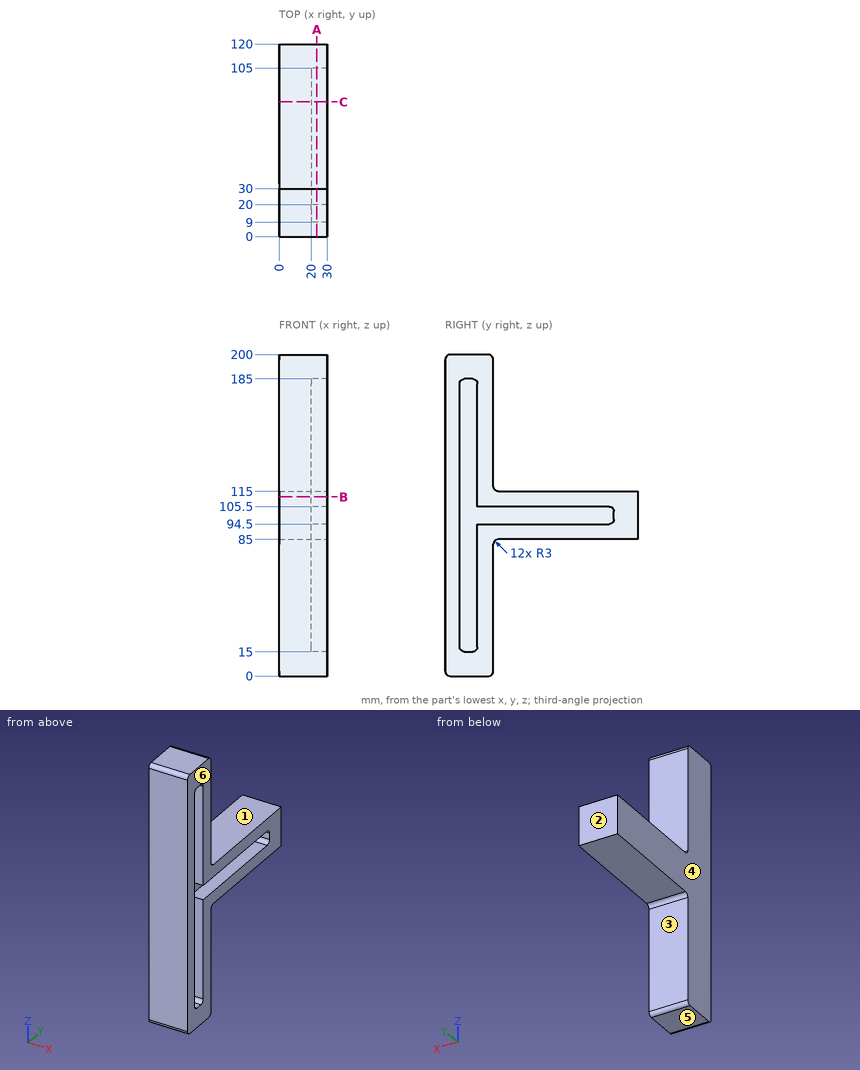
Check sheet for the drawn part. Datum: minimum x, y, z corner. Units: mm. A direction names the side the tool comes from. Round coordinates to 2 decimals unless told otherwise and drop trailing zeros. Loops run counter-clockwise (first coordinate to the right, second up) from the corner with the lowest first, then second, coordinate; pieces in that order, holes last. Notation, with made-up numbers: (12, 7) - (46, 7) arc R38 cw to (46, 45) - close; hole circle Ø3 at (77.25, 86.5). An arc over 180 degrees is marked (long way). Answer as a JSON object with one key per item and string values. Group by question number.
Q1. Sectioned sample at B-B, the plane z = 111.5. Enter the section's corners in (x, y).
Q2. Sectioned sample at C-C, the plane y = 84. Enter the section's corners in (x, z), plus the area to 3 significant figures.
Q3. Scan lines: line 1 along Z through (x, y) = (25, 77); line 2 along Y through (x, z) = (23.5, 141); line 3 along Y through (x, z) = (21.5, 85.5). Record each from-to range of solid material in increasing order. Write a range as [from, to].
Q4. Gauge pin test, flat ends, axial feed: P1, Ø8, axis at x = 26, y = 80.5, coming from the +Z side; P2, Ø8, axis at x = 23.5, z = 139.5, coming from the +Y side; P3, Ø5, axis at x = 21, y = 40, coming from the -Z side; P4, Ø1.5, axis at y = 96, z = 94.5, coming from the -X side. Record the tip position at first contact, or that the pin passes through.
Q5. Set-up check for the marked faces 1, 2 and 3: record each of +Z, -Z, +X, -X, +Y, -Y from which the full face is reachable in a straight line by a thin tool's end or side.
Q6. Mould release check, pull along X, two halves, no side actions. Record for the marked faces 4, 5 and 6: released by +X, released by -X, zero draft, split by the parting line, or undercut.
Q7. Sectioned sample at A-A, the plane x = 23.5. Enter the section's corners in (y, z), plus the area to 3 significant figures.
Solution:
{
 "1": {"outline": "(0, 0) - (30, 0) - (30, 9) - (20, 9) - (20, 20) - (30, 20) - (30, 120) - (0, 120) - close"},
 "2": {"outline": "(0, 85) - (30, 85) - (30, 94.5) - (20, 94.5) - (20, 105.5) - (30, 105.5) - (30, 115) - (0, 115) - close", "area": "790 mm²"},
 "3": {"line 1": "z = [85, 94.5], [105.5, 115]", "line 2": "y = [0, 9], [20, 30]", "line 3": "y = [0, 9], [20, 120]"},
 "4": {"P1": "stops at z = 115", "P2": "stops at y = 30", "P3": "stops at z = 85", "P4": "stops at x = 0"},
 "5": {"face 1": "+Z, +X, -X, +Y", "face 2": "+Z, -Z, +X, -X, +Y", "face 3": "-Z, +X, -X, +Y"},
 "6": {"face 4": "released by -X", "face 5": "zero draft", "face 6": "released by +X"},
 "7": {"outline": "(0, 3) arc R3 ccw to (3, 0) - (27, 0) arc R3 ccw to (30, 3) - (30, 82) arc R3 cw to (33, 85) - (120, 85) - (120, 115) - (33, 115) arc R3 cw to (30, 118) - (30, 197) arc R3 ccw to (27, 200) - (3, 200) arc R3 ccw to (0, 197) - close; hole (9, 18) arc R3 ccw to (12, 15) - (17, 15) arc R3 ccw to (20, 18) - (20, 94.5) - (102, 94.5) arc R3 ccw to (105, 97.5) - (105, 102.5) arc R3 ccw to (102, 105.5) - (20, 105.5) - (20, 182) arc R3 ccw to (17, 185) - (12, 185) arc R3 ccw to (9, 182) - close", "area": "5,900 mm²"}
}
